Geometry check sheet. Reference: the model listing, model coordinates, mm. A direction names the side the tool comes from. Coordinates: 2 decimals unless noted, no trailing zeros.
Autodesk Inventor part; units mm, degrees
ref_plane "Plan YZ" through (0, 0, 0) normal (1, 0, 0) x (0, 1, 0)
ref_plane "Plan XZ" through (0, 0, 0) normal (0, 1, 0) x (-1, 0, 0)
ref_plane "Plan XY" through (0, 0, 0) normal (0, 0, 1) x (1, 0, 0)
sketch "Esquisse1" plane through (0, 0, 0) normal (0, 0, 1) x (1, 0, 0)
  line L0 (0, 11.8) -> (0, 0)
  ellipse E0 centre (0, 5.9) end of major axis (14.65, 5.9) minor radius 5.9
  dimension "d13" = 14.65
  dimension "d1" = 11.8
extrude "Extrusion3" add sketch "Esquisse1" along normal blind 0.8 contours E0 L0 picked at (3.5971, 4.141)
sketch "Esquisse7" plane through (0, 0, 0.8) normal (0, 0, 1) x (1, 0, 0)
  ellipse E0 centre (0.7, 5.9) end of major axis (13.95, 5.9) minor radius 5.2
  line L0 (0.7, 11.1) -> (0.7, 0.7)
  line L1 (0, 11.8) -> (0, 0)
  line L2 (0.7, 11.7933) -> (0.7, 11.1) construction
  line L3 (0.7, 0.7) -> (0.7, 0.0067) construction
  ellipse E1 centre (0, 5.9) end of major axis (14.65, 5.9) minor radius 5.9 (0, 0) -> (0, 11.8) ccw
  dimension "d16" = 13.25
  dimension "d17" = 10.4
  dimension "d18" = 0.7
extrude "Extrusion4" add sketch "Esquisse7" along normal blind 6.7 contours E0 L0
sketch "Esquisse8" plane through (0, 0, 0) normal (0, 0, -1) x (-1, 0, 0)
  circle A0 centre (-6, 5.9) radius 4.3
  line L0 (0, 11.8) -> (0, 0)
  line L1 (2.2688, 5.9) -> (-1.7595, 5.9) construction
  line L2 (0, 0) -> (0, 5.9) construction
  line L3 (0, 5.9) -> (0, 11.8) construction
  line L4 (-0.7, 0.7) -> (-0.7, 11.1) construction
  dimension "d21" = 8.6
  dimension "d26" = 5.3
extrude "Extrusion5" cut sketch "Esquisse8" against normal blind 3
properties part number "P1704_019_button_triangle_cap" material "."
(1) Scan lines: L1, parallel to Z at x = 3.25, y = 8.5; L2, parallel to Y at x = 6, z = 1.05; L3, parallel to Y at x = 9.75, z = 2.25. Record each from-to range of solid material in increasing order.
Findings:
L1: z = 3 to 7.5
L2: y = 1.13 to 1.6, 10.2 to 10.67
L3: y = 2.1 to 3.8, 8 to 9.7
(2) Access from +Z, -Z, +X, -X, +Y, -Y to the whole of each face (thin tool, end or side, straight path). Record for faces 3 (the flat face through (0.7, 6, 4)), 4 (the flat face through (6, 6, 7.5)), 5 (the flat face through (6, 6, 3)).
Findings:
face 3: +Z, -X, +Y, -Y
face 4: +Z, +X, -X, +Y, -Y
face 5: -Z
(3) Gauge pin test, flat ends, axial feed: pin 1 Ø3 at (y, z) = (4.5, 4) entering from -X; pin 2 Ø4 at (y, z) = (3, 6.5) entering from +X. Record the tip position at first contact, or that the pin passes through.
Findings:
pin 1: stops at x = 0.7
pin 2: stops at x = 13.75
(4) Draft check along Y on faces 1 (the flat face through (6.7, 10.7, 0.8)), 2 (the cylindrical face through (9.41, 3.28, 1.48)). Enter one of: +Y half, -Y half, draft (parallel to the pull), parting line (faces both ways), or undercut.
Findings:
face 1: draft
face 2: undercut
